Read the model definition and answer for the solid it produces. Units are mm, in the model's axes. Round coordinates to 2 decimals unless told otherwise and drop trailing zeros. Loops run counter-clockwise (first coordinate to the right, second up) from the corner with the lowest first, then second, coordinate; pieces in that order, holes last. Notation, with made-up numbers: M 23,84.5 L 42,84.5 A16 cw 42,108.5 Z; hole C -3,27 d3. An arc over 180 degrees is marked long. Answer as CSV lines item,"result".
```python
from build123d import *

# Parameters (mm, degrees)
ESQUISSE5_R             = 1.75
ENL_V_MAT_EXTRU_3_DEPTH = 10


with BuildPart() as part:
    # Esquisse1 → Révolution1 (revolve)
    with BuildSketch(Plane(origin=(0, 0, 0), x_dir=(0, 0, -1), z_dir=(1, 0, 0)), mode=Mode.PRIVATE) as r_volution1_sk:
        Polygon((101.754375518, 10), (101.754375518, 7.872703136), (102.754375518, 7.872703136), (102.754375518, 10), (113.254375518, 10), (113.254375518, 5), (115.25030387, 5), (115.25030387, 10), (120.254297163, 10), (120.254297163, 0), (0.004375518, 0), (0.004375518, 10), align=None)
    revolve(r_volution1_sk.sketch.rotate(Axis((0, 10, -0.004375518), (0, -1, 0)), 180), axis=Axis((0, 10, -0.004375518), (0, -1, 0)))

    # Esquisse5 → Enlèv. mat.-Extru.3 (cut)
    with BuildSketch(Plane.XZ):
        with Locations(Location((-65, 65, 0), (0, 0, 270))):
            Circle(ESQUISSE5_R)
        with Locations(Location((-65, -65, 0), (0, 0, 270))):
            Circle(ESQUISSE5_R)
        with Locations(Location((65, 65, 0), (0, 0, 270))):
            Circle(ESQUISSE5_R)
        with Locations(Location((65, -65, 0), (0, 0, 270))):
            Circle(ESQUISSE5_R)
    extrude(amount=-ENL_V_MAT_EXTRU_3_DEPTH, mode=Mode.SUBTRACT)


solid = part.part
```
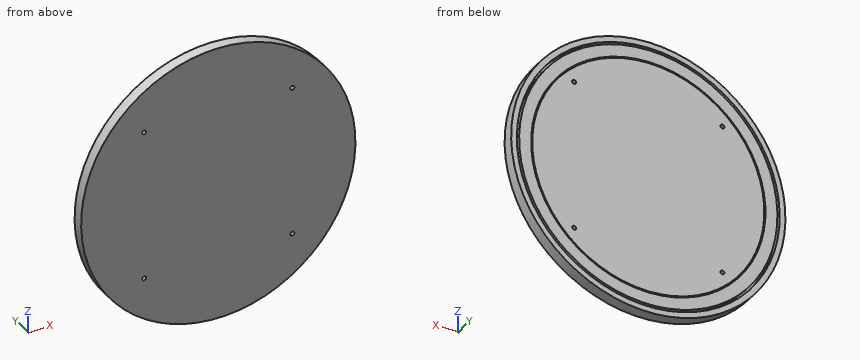
1) Find section B-B, the plane z = -45. Give the vertices of the cut face in (x, y).
Evaluation:
outline,"M -111.51,0 L 111.51,0 L 111.51,10 L 106.1,10 L 106.1,5 L 103.93,5 L 103.93,10 L 92.37,10 L 92.37,7.87 L 91.26,7.87 L 91.26,10 L -91.26,10 L -91.26,7.87 L -92.37,7.87 L -92.37,10 L -103.93,10 L -103.93,5 L -106.1,5 L -106.1,10 L -111.51,10 Z"
2) Find section A-A, the plane y = 3. Give the vertices of the cut face in (x, z), then the cut area to 3 significant figures.
Evaluation:
outline,"C 0,0 d240.5; hole C -65,-65 d3.5; hole C -65,65 d3.5; hole C 65,-65 d3.5; hole C 65,65 d3.5"
area,"45,400 mm^2"
3) Each of these flat-tipped pins is pushed along its axis until it touches: P1, Ø3, axis at x = 65, z = 65, coming from the +Y side; P2, Ø5, axis at x = 59, y = 2, coming from the +Z side; P3, Ø2, axis at y = 7, z = -18, coming from the -X side; P4, Ø4, axis at x = 61.5, y = 6.5, coming from the +Z side. Where does it stop, or does it pass through?
Evaluation:
P1,"passes through"
P2,"stops at z = 106.15"
P3,"stops at x = -119.04"
P4,"stops at z = 104.49"
4) Find section C-C, the plane x = -73. Give the vertices of the cut face in (y, z) (3 decimals).
Evaluation:
outline,"M 0,-95.561 L 10,-95.561 L 10,-89.182 L 5,-89.182 L 5,-86.587 L 10,-86.587 L 10,-72.313 L 7.873,-72.313 L 7.873,-70.885 L 10,-70.885 L 10,70.876 L 7.873,70.876 L 7.873,72.304 L 10,72.304 L 10,86.578 L 5,86.578 L 5,89.173 L 10,89.173 L 10,95.552 L 0,95.552 Z"
5) Straight lines are drawn through the part: line 1 (Z direction, x = -1, y = 8.5); line 2 (Z direction, x = 83.5, y = 5.25); line 3 (X direction, y = 2.5, z = 65). For each, find the intervals that lie inside material, in ascending order.
Evaluation:
line 1,"z = -120.25 to -115.25, -113.25 to -102.75, -101.75 to 101.74, 102.74 to 113.24, 115.24 to 120.24"
line 2,"z = -86.54 to -79.44, -76.51 to 76.5, 79.43 to 86.53"
line 3,"x = -101.17 to -66.75, -63.25 to 63.25, 66.75 to 101.17"
6) Find section D-D, the plane x = 106.5. Give the vertices of the cut face in (y, z), then the cut area to 3 significant figures.
Evaluation:
outline,"M 0,-55.84 L 10,-55.84 L 10,-44.04 L 5,-44.04 L 5,-38.52 L 10,-38.52 L 10,38.51 L 5,38.51 L 5,44.03 L 10,44.03 L 10,55.83 L 0,55.83 Z"
area,"1,060 mm^2"
